```python
from build123d import *

# Parameters (mm, degrees)
SKETCH094_R             = 12.2
PAD046_DEPTH            = 30
SKETCH095_R             = 3.2
PAD042_DEPTH            = 1.4
SKETCH100_R             = 1
PAD045_DEPTH            = 8
SKETCH098_R             = 11.95
POCKET040_DEPTH         = 1
SKETCH096_R             = 3.2
PAD047_DEPTH            = 2.2
SKETCH099_R             = 1
PAD044_DEPTH            = 2.7
SKETCH097_W             = 0.7
SKETCH097_H             = 2.8
PAD043_DEPTH            = 6
FILLET018_R             = 1
BODY016_PITCH_ANGLE     = 90
BODY016_PLACEMENT_ANGLE = -90


with BuildPart() as part:
    # Sketch094 → Pad046 (new body)
    with BuildSketch(Plane.XY):
        Circle(SKETCH094_R)
    extrude(amount=PAD046_DEPTH)

    # Sketch095 (on Face3 of Pad046) → Pad042 (join)
    with BuildSketch(Plane.XY.offset(30)):
        Circle(SKETCH095_R)
    extrude(amount=PAD042_DEPTH)

    # Sketch100 (on Face5 of Pad042) → Pad045 (join)
    with BuildSketch(Plane.XY.offset(31.4)):
        Circle(SKETCH100_R)
    extrude(amount=PAD045_DEPTH)

    # Sketch098 (on Face2 of Pad045) → Pocket040 (cut)
    with BuildSketch(Plane(origin=(0, 0, 0), x_dir=(1, 0, 0), z_dir=(0, 0, -1))):
        Circle(SKETCH098_R)
    extrude(amount=-POCKET040_DEPTH, mode=Mode.SUBTRACT)

    # Sketch096 (on Face6 of Pocket040) → Pad047 (join)
    with BuildSketch(Plane(origin=(0, 0, 1), x_dir=(1, 0, 0), z_dir=(0, 0, -1))):
        Circle(SKETCH096_R)
    extrude(amount=PAD047_DEPTH)

    # Sketch099 (on Face10 of Pad047) → Pad044 (join)
    with BuildSketch(Plane(origin=(0, 0, -1.2), x_dir=(1, 0, 0), z_dir=(0, 0, -1))):
        Circle(SKETCH099_R)
    extrude(amount=PAD044_DEPTH)

    # Sketch097 (on Face6 of Pad044) → Pad043 (join)
    with BuildSketch(Plane(origin=(0, 0, 1), x_dir=(1, 0, 0), z_dir=(0, 0, -1))):
        with Locations((-8.65, 0)):
            Rectangle(SKETCH097_W, SKETCH097_H)
        with Locations((8.65, 0)):
            Rectangle(SKETCH097_W, SKETCH097_H)
    extrude(amount=PAD043_DEPTH)

    # Fillet018
    fillet018_edges = [part.edges().sort_by_distance(p)[0] for p in [
        (-8.65, -1.4, -5),
        (-8.65, 1.4, -5),
        (8.65, -1.4, -5),
        (8.65, 1.4, -5),
    ]]
    fillet(fillet018_edges, radius=FILLET018_R)


with BuildPart() as part_1:
    # Body016 pitch: moved
    add(part.part.rotate(Axis((0, 0, 0), (0, 1, 0)), BODY016_PITCH_ANGLE))


with BuildPart() as part_2:
    # Body016 placement: moved
    add(part_1.part.moved(Location((15, 0, 22))).rotate(Axis((15, 0, 22), (0, 0, 1)), BODY016_PLACEMENT_ANGLE))


solid = part_2.part
```
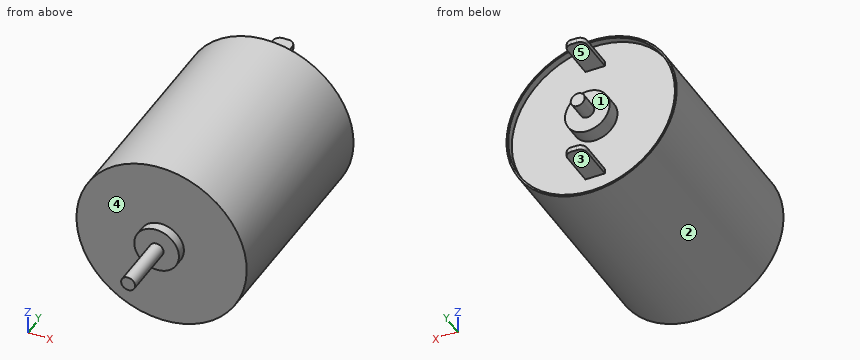
For this review, take the finished solid that the model builds, in its own axes (mm). Face numbers are marked on the shaded views. A direction names the side the tool comes from. Round coordinates to 2 decimals unless told otherwise and drop trailing zeros. Write each loop counter-clockwise with the first axis right and the second up, starting at its lowest first coordinate (ties: lowest second). Pieces come first, ordered by that corner, then holes.
1) Mouldability with a two-part tool opening along X and no side actions: class the marked faces 1, 2 and 3 as +X half, -X half, draft (parallel to the pull), parting line (faces both ways), or undercut.
Answer below:
face 1: draft
face 2: parting line
face 3: undercut
2) Machinability: for the marked faces 4 and 5, which of the approach directions +Z, -Z, +X, -X, +Y, -Y give a long, thin tool a straight path to every point of the face, cutting with its end or side? Answer none if there is none.
Answer below:
face 4: -Y
face 5: +Y
3) Take a section at D-D on z = 17. Give the boundary of the cut face in (x, y), then the cut area to 3 significant figures.
Answer below:
outline: (3.87, -30) - (26.13, -30) - (26.13, 0) - (25.85, 0) - (25.85, -1) - (4.15, -1) - (4.15, 0) - (3.87, 0) - close
area: 646 mm2
4) For line 1 along X through (y, z) = (-0.65, 22); line 2 along Y through (x, z) = (20.25, 17.25); line 3 along X through (y, z) = (-0.5, 32.5), list the stretches that pass through material, from the lowest coordinate up.
Answer below:
line 1: x = 2.8 to 3.05, 11.8 to 18.2, 26.95 to 27.2
line 2: y = -30 to -1
line 3: x = 8.79 to 9.29, 20.71 to 21.21
5) Insertion check: pin 1 Ø10 at (x, z) = (12, 24) entering from +Y; pin 2 Ø1.4 at (x, y) = (14.5, 3) entering from +Z; pin 3 Ø3 at (x, y) = (15, 1) entering from -Z; pin 4 Ø3 at (x, z) = (6, 14.5) entering from -Y. Each pin has a flat end and moves straight along its axis. Give the tip position at first contact, or say it passes through.
Answer below:
pin 1: stops at y = 3.9
pin 2: stops at z = 31
pin 3: stops at z = 9.8
pin 4: stops at y = -30
6) Take a section at C-C on x = 21. Give the boundary of the cut face in (y, z).
Answer below:
outline: (-30, 11.38) - (0, 11.38) - (0, 11.67) - (-1, 11.67) - (-1, 32.33) - (0, 32.33) - (0, 32.62) - (-30, 32.62) - close
7) Take a section at A-A on z = 22. Give the boundary of the cut face in (x, y), then the cut area to 3 significant figures.
Answer below:
outline: (2.8, -30) - (11.8, -30) - (11.8, -31.4) - (14, -31.4) - (14, -39.4) - (16, -39.4) - (16, -31.4) - (18.2, -31.4) - (18.2, -30) - (27.2, -30) - (27.2, 0) - (26.95, 0) - (26.95, -1) - (18.2, -1) - (18.2, 1.2) - (16, 1.2) - (16, 3.9) - (14, 3.9) - (14, 1.2) - (11.8, 1.2) - (11.8, -1) - (3.05, -1) - (3.05, 0) - (2.8, 0) - close
area: 753 mm2
8) Take a section at B-B on y = -29. Give the boundary of the cut face in (x, z), then the cut area to 3 significant figures.
Answer below:
outline: circle Ø24.4 at (15, 22)
area: 468 mm2
